Check sheet for the drawn part. Datum: minimum x, y, z corner. Units: mm. Give positions to 0.01 mm unless a question says otherwise; leave off trailing zeros. Loops run counter-clockwise (first coordinate to the right, second up) from the corner with the lowest first, then second, coordinate; pieces in that order, holes last.
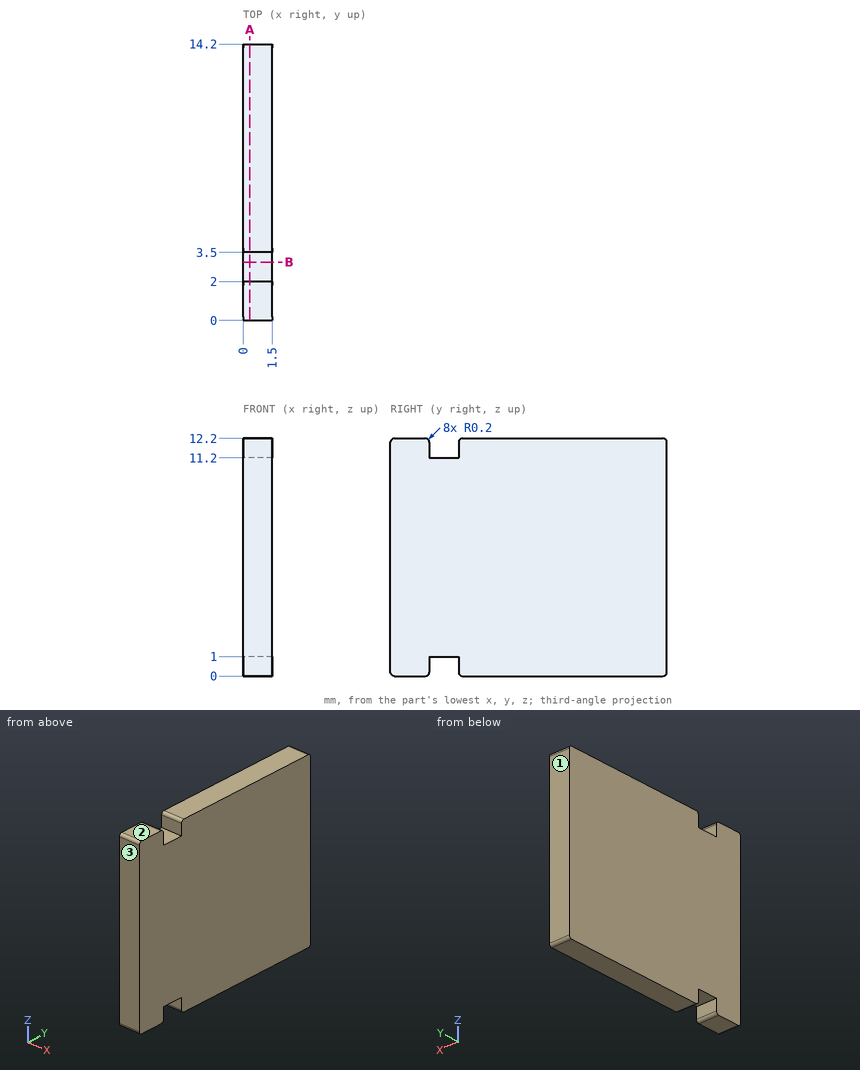
1) Sectioned sample at B-B on y = 3. Enter the section's corners in (x, z), plus the area to 3 significant figures.
2) Sectioned sample at A-A on x = 0.35. Enter the section's corners in (y, z), plus the area to 3 significant figures.
3) Depth check by flat-ended pin: P1, Ø0.8, axis at x = 0.5, y = 2.5, coming from the +Z side. Enter the tip coordinate at first touch or a pass-through.
4) Mould release check, pull along Y, two halves, no side actions. Record for the marked faces 1, 2 and 3: +Y half, -Y half, draft (parallel to the pull), parting line (faces both ways), or undercut.
5) Scan line: line 1 along Y through (x, z) = (0.4, 11.5). Record every from-to range of solid material in increasing order.
Determined:
1. outline: (0, 1) - (1.5, 1) - (1.5, 11.2) - (0, 11.2) - close
1. area: 15.3 mm2
2. outline: (0, 0.2) arc R0.2 ccw to (0.2, 0) - (1.8, 0) arc R0.2 ccw to (2, 0.2) - (2, 1) - (3.5, 1) - (3.5, 0.2) arc R0.2 ccw to (3.7, 0) - (14, 0) arc R0.2 ccw to (14.2, 0.2) - (14.2, 12) arc R0.2 ccw to (14, 12.2) - (3.7, 12.2) arc R0.2 ccw to (3.5, 12) - (3.5, 11.2) - (2, 11.2) - (2, 12) arc R0.2 ccw to (1.8, 12.2) - (0.2, 12.2) arc R0.2 ccw to (0, 12) - close
2. area: 170 mm2
3. P1: stops at z = 11.2
4. face 1: +Y half
4. face 2: draft
4. face 3: -Y half
5. line 1: y = 0 to 2, 3.5 to 14.2
